from build123d import *

# Parameters (mm, degrees)
SKETCH_1_R          = 4.15
EXTRUDE_1_DEPTH     = 4
FILLET_1_R          = 50
SKETCH_4_R          = 5
EXTRUDE_2_DEPTH     = 5
SKETCH_5_R          = 6
EXTRUDE_3_DEPTH     = 0.5
SKETCH_6_R          = 3.15
CUT_EXTRUDE_2_DEPTH = 3
SKETCH_7_R          = 1.85
CUT_EXTRUDE_3_DEPTH = 10
SKETCH_8_R          = 5.2
CUT_EXTRUDE_4_DEPTH = 1


with BuildPart() as part:
    # 草图1 → 凸台-拉伸1 (new body)
    with BuildSketch(Plane.XY):
        with BuildLine():
            Line((-5.999958142, -11.451976213), (-5.999958142, -41.451976213))
            ThreePointArc((-5.999958142, -41.451976213), (-1.999958142, -53.075451596), (2.000041858, -41.451976213))
            Line((2.000041858, -41.451976213), (2.000041858, -11.451976213))
            ThreePointArc((2.000041858, -11.451976213), (-1.999958142, 0.17149917), (-5.999958142, -11.451976213))
        make_face()
        with Locations(Location((-1.999958142, -6.32850083, 0), (0, 0, 180))):
            Circle(SKETCH_1_R, mode=Mode.SUBTRACT)
    extrude(amount=EXTRUDE_1_DEPTH)

    # 圆角1
    fillet_1_edges = [part.edges().sort_by_distance(p)[0] for p in [
        (-5.999958142, -41.451976213, 2),
        (-5.999958142, -11.451976213, 2),
        (2.000041858, -11.451976213, 2),
        (2.000041858, -41.451976213, 2),
    ]]
    fillet(fillet_1_edges, radius=FILLET_1_R)

    # 草图4 → 凸台-拉伸2 (add)
    with BuildSketch(Plane(origin=(0, 0, 0), x_dir=(-1, 0, 0), z_dir=(0, 0, -1))):
        with Locations((1.999958142, -46.575451596)):
            Circle(SKETCH_4_R)
    extrude(amount=EXTRUDE_2_DEPTH)

    # 草图5 → 凸台-拉伸3 (add)
    with BuildSketch(Plane(origin=(0, 0, 0), x_dir=(-1, 0, 0), z_dir=(0, 0, -1))):
        with Locations((1.999958142, -46.575451596)):
            Circle(SKETCH_5_R)
    extrude(amount=EXTRUDE_3_DEPTH)

    # 草图6 → 切除-拉伸2 (cut)
    with BuildSketch(Plane(origin=(0, 0, -5), x_dir=(-1, 0, 0), z_dir=(0, 0, -1))):
        with Locations((1.999958142, -46.575451596)):
            Circle(SKETCH_6_R)
    extrude(amount=-CUT_EXTRUDE_2_DEPTH, mode=Mode.SUBTRACT)

    # 草图7 → 切除-拉伸3 (cut)
    with BuildSketch(Plane(origin=(0, 0, -2), x_dir=(-1, 0, 0), z_dir=(0, 0, -1))):
        with Locations((1.999958142, -46.575451596)):
            Circle(SKETCH_7_R)
    extrude(amount=-CUT_EXTRUDE_3_DEPTH, mode=Mode.SUBTRACT)

    # 草图8 → 切除-拉伸4 (cut)
    with BuildSketch(Plane.XY.offset(4)):
        with Locations((-1.999958142, -6.32850083)):
            Circle(SKETCH_8_R)
    extrude(amount=-CUT_EXTRUDE_4_DEPTH, mode=Mode.SUBTRACT)


solid = part.part
Model file for the job. Use its own axes, mm. A direction names the side the tool comes from. Round coordinates to 2 decimals unless told otherwise and drop trailing zeros. Order: outer loops, then holes, each group sorted by start corner. A loop starts at its lowest first (then second) coordinate and runs counter-clockwise, first axis right, second up.
(1) Band-saw the part on D-D (z = 1). List the corners of the cut face in (x, y), then the cut area to 3 significant figures.
(2) Pin check, flat tips, straight feed: pin 1 (5 mm diameter, centred on y = -35.5, z = 0, fed in from +X); pin 2 (3.5 mm diameter, centred on x = -2, y = -46.58, fed in from -Z); pin 3 (6.5 mm diameter, centred on x = -3.5, y = -22.5, fed in from -Z); pin 4 (5 mm diameter, centred on x = -2, y = -46.58, fed in from -Z). Stop position of each tip, or through.
(3) Band-saw the part on C-C (x = 0.5). List the corners of the cut face in (y, z).
(4) 3-axis set-ups, long thin cutter, end or side, ignore diameter. For faces 5 (the face through (-1.32, -49.65, -3.52)), 6 (the face through (-2.85, -48.22, 0.96)), 7 (the face through (2.572, -37.495, 2.028)), 8 (the face through (-6, -26, 2)): which of +Z, -Z, +X, -X, +Y, -Y reach the whole face in a straight line?
(5) Pull direction X, two halves, no side cores. Call faces 1 (the face through (0.4, -10.94, 3.51)), 2 (the face through (-2, -20, 0)), 3 (the face through (2.57, -15.41, 2.03)), 4 (the face through (-6, -8, 3)): released by +X, released by -X, zero draft, split by the parting line, or undercut.
(6) Drill centre lines: line 1 (Y direction, x = -1.25, z = 3.25); line 2 (Z direction, x = -6.5, y = -7); line 3 (Y direction, x = 1, z = 0.5). Where is each one in solid material? Low to high.
(7) Band-saw the part on B-B (x = -2.5). List the corners of the cut face in (y, z).
(8) Band-saw the part on A-A (y = -7). List the corners of the cut face in (x, z), then the cut area to 3 significant figures.
Verdict:
1. outline: (-8.21, -44.66) arc R6.5 ccw (long way) to (4.21, -44.66) arc R50 cw to (2, -29.95) - (2, -22.95) arc R50 cw to (4.21, -8.24) arc R6.5 ccw (long way) to (-8.21, -8.24) arc R50 cw to (-6, -22.95) - (-6, -29.95) arc R50 cw to start; hole circle Ø8.3 at (-2, -6.33); hole circle Ø3.7 at (-2, -46.58)
1. area: 451 mm2
2. pin 1: stops at x = 2.65
2. pin 2: passes through
2. pin 3: stops at z = 0
2. pin 4: stops at z = -2
3. outline: (-52.58, 0) - (-52.03, 0) - (-52.03, -0.5) - (-50.91, -0.5) - (-50.91, -5) - (-48.49, -5) - (-48.49, -2) - (-44.66, -2) - (-44.66, -5) - (-42.25, -5) - (-42.25, -0.5) - (-41.12, -0.5) - (-41.12, 0) - (-9.64, 0) - (-9.64, 3) - (-10.89, 3) - (-10.89, 4) - (-52.58, 4) - close; (-3.02, 0) - (-0.33, 0) - (-0.33, 4) - (-1.77, 4) - (-1.77, 3) - (-3.02, 3) - close
4. face 5: -Z
4. face 6: +Z, -Z
4. face 7: +Z, -Z, +X
4. face 8: +Z, -Z, -X
5. face 1: undercut
5. face 2: zero draft
5. face 3: released by +X
5. face 4: undercut
6. line 1: y = -53.03 to -48.27, -44.88 to -11.47, -1.18 to 0.13
6. line 2: z = 0 to 3
6. line 3: y = -52.34 to -9.2, -3.46 to -0.56
7. outline: (-53.06, 0) - (-52.55, 0) - (-52.55, -0.5) - (-51.55, -0.5) - (-51.55, -5) - (-49.69, -5) - (-49.69, -2) - (-48.36, -2) - (-48.36, 4) - (-53.06, 4) - close; (-44.79, -2) - (-43.47, -2) - (-43.47, -5) - (-41.6, -5) - (-41.6, -0.5) - (-40.6, -0.5) - (-40.6, 0) - (-10.45, 0) - (-10.45, 3) - (-11.5, 3) - (-11.5, 4) - (-44.79, 4) - close; (-2.21, 0) - (0.15, 0) - (0.15, 4) - (-1.15, 4) - (-1.15, 3) - (-2.21, 3) - close
8. outline: (-8.47, 0) - (-6.1, 0) - (-6.1, 3) - (-7.16, 3) - (-7.16, 4) - (-8.47, 4) - close; (2.1, 0) - (4.47, 0) - (4.47, 4) - (3.16, 4) - (3.16, 3) - (2.1, 3) - close
8. area: 16.8 mm2
